Part model, mm, in its own coordinate system. Face numbers are marked on the shaded views. Round coordinates to 2 decimals unless told otherwise and drop trailing zeros. Write each loop counter-clockwise with the first axis right and the second up, starting at its lowest first coordinate (ties: lowest second). Pieces come first, ordered by that corner, then holes.
```python
from build123d import *

# Parameters (mm, degrees)
SKETCH_1_W          = 72
SKETCH_1_H          = 99.6
SKETCH_1_R          = 1.6
EXTRUDE_1_DEPTH     = 2
FILLET_1_R          = 3
SKETCH_7_W          = 2.173613934
SKETCH_7_H          = 4.368539476
CUT_EXTRUDE_1_DEPTH = 10
CUT_EXTRUDE_2_DEPTH = 10
FILLET_2_R          = 2
SKETCH_9_W          = 2.173613934
SKETCH_9_H          = 2.184269738
EXTRUDE_5_DEPTH     = 2
FILLET_4_R          = 2
FILLET_5_R          = 2
EXTRUDE_4_DEPTH     = 5


with BuildPart() as part:
    # Sketch 1 → Extrude 1 (new body)
    with BuildSketch(Plane(origin=(0, 0, 0), x_dir=(1, 0, 0), z_dir=(0, 1, 0))):
        with Locations((36, -49.8)):
            Rectangle(SKETCH_1_W, SKETCH_1_H)
        with Locations(Location((11, -5, 0), (0, 0, 270))):
            Circle(SKETCH_1_R, mode=Mode.SUBTRACT)
        with Locations(Location((14, -95, 0), (0, 0, 270))):
            Circle(SKETCH_1_R, mode=Mode.SUBTRACT)
        with Locations(Location((58, -95, 0), (0, 0, 90))):
            Circle(SKETCH_1_R, mode=Mode.SUBTRACT)
        with Locations(Location((61, -5, 0), (0, 0, 90))):
            Circle(SKETCH_1_R, mode=Mode.SUBTRACT)
        with Locations(Location((2.31, -58.92, 0), (0, 0, 270))):
            Circle(SKETCH_1_R, mode=Mode.SUBTRACT)
        with Locations(Location((69.69, -58.92, 0), (0, 0, 90))):
            Circle(SKETCH_1_R, mode=Mode.SUBTRACT)
    extrude(amount=EXTRUDE_1_DEPTH)

    # Fillet 1
    fillet_1_edges = [part.edges().sort_by_distance(p)[0] for p in [
        (0, 1, 0),
        (72, 1, 0),
        (72, 1, 99.6),
        (0, 1, 99.6),
    ]]
    fillet(fillet_1_edges, radius=FILLET_1_R)

    # Sketch 7 → Cut-Extrude 1 (cut)
    with BuildSketch(Plane(origin=(0, 2, 0), x_dir=(1, 0, 0), z_dir=(0, 1, 0))):
        with Locations((36, -99.6)):
            Rectangle(SKETCH_7_W, SKETCH_7_H)
    extrude(amount=-CUT_EXTRUDE_1_DEPTH, mode=Mode.SUBTRACT)

    # Sketch 8 → Cut-Extrude 2 (cut)
    with BuildSketch(Plane(origin=(0, 2, 0), x_dir=(1, 0, 0), z_dir=(0, 1, 0))):
        with BuildLine():
            Line((3, -99.6), (3, -79.6))
            Line((3, -79.6), (0, -79.6))
            Line((0, -79.6), (0, -96.6))
            ThreePointArc((0, -96.6), (0.878679656, -98.721320344), (3, -99.6))
        make_face()
        with BuildLine():
            ThreePointArc((72, -96.6), (71.121320344, -98.721320344), (69, -99.6))
            Line((69, -99.6), (69, -79.6))
            Line((69, -79.6), (72, -79.6))
            Line((72, -79.6), (72, -96.6))
        make_face()
        with BuildLine():
            ThreePointArc((3, 0), (0.878679656, -0.878679656), (0, -3))
            Line((0, -3), (0, -18))
            Line((0, -18), (3, -18))
            Line((3, -18), (3, 0))
        make_face()
    cut_extrude_2 = extrude(amount=-CUT_EXTRUDE_2_DEPTH, mode=Mode.SUBTRACT)

    # Fillet 2
    fillet_2_edges = [part.edges().sort_by_distance(p)[0] for p in [
        (69, 1, 79.6),
        (3, 1, 79.6),
    ]]
    fillet(fillet_2_edges, radius=FILLET_2_R)

    # Mirror 2: Cut-Extrude 2 across plane
    add(cut_extrude_2.mirror(Plane(origin=(36, 0, 0), x_dir=(0, 0, 1), z_dir=(1, 0, 0))), mode=Mode.SUBTRACT)

    # Sketch 9 → Extrude 5 (add)
    with BuildSketch(Plane(origin=(0, 2, 0), x_dir=(1, 0, 0), z_dir=(0, 1, 0))):
        with Locations((36, -98.507865131)):
            Rectangle(SKETCH_9_W, SKETCH_9_H)
    extrude(amount=-EXTRUDE_5_DEPTH)

    # Fillet 4
    fillet_4_edges = [part.edges().sort_by_distance(p)[0] for p in [
        (69, 1, 18),
        (3, 1, 18),
    ]]
    fillet(fillet_4_edges, radius=FILLET_4_R)

    # Fillet 5
    fillet_5_edges = [part.edges().sort_by_distance(p)[0] for p in [
        (3, 1, 79.6),
        (69, 1, 79.6),
    ]]
    fillet(fillet_5_edges, radius=FILLET_5_R)


with BuildPart() as body_2:
    # Sketch 6 → Extrude 4 (new body)
    with BuildSketch(Plane(origin=(0, -3, 0), x_dir=(-1, 0, 0), z_dir=(0, -1, 0))):
        with BuildLine():
            Line((-2, 4), (-70, 4))
            ThreePointArc((-70, 4), (-74.242640687, 2.242640687), (-76, -2))
            Line((-76, -2), (-76, -18))
            Line((-76, -18), (-76, -97.6))
            ThreePointArc((-76, -97.6), (-74.242640687, -101.842640687), (-70, -103.6))
            Line((-70, -103.6), (-2, -103.6))
            ThreePointArc((-2, -103.6), (2.242640687, -101.842640687), (4, -97.6))
            Line((4, -97.6), (4, -4))
            ThreePointArc((4, -4), (3.146700168, 1.610025126), (-2, 4))
        make_face()
    extrude(amount=-EXTRUDE_4_DEPTH)

    # Combine 1: cut part
    add(part.part, mode=Mode.SUBTRACT)


solid = body_2.part
```
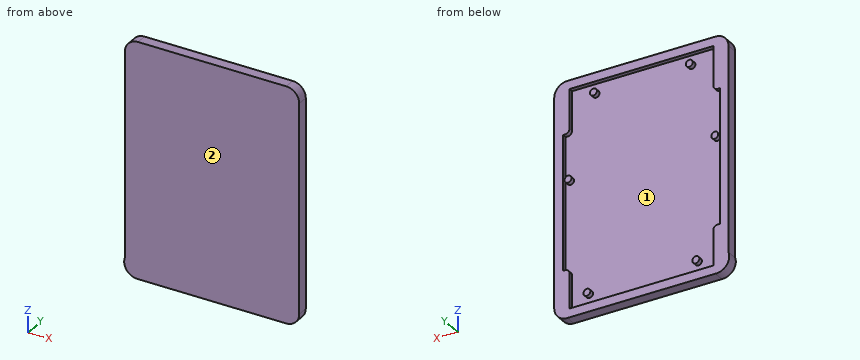
Q1. Cut at C-C on x = 14. Write the cut outline in (y, z), plus the area to 3 significant figures.
Values follow:
outline: (-3, -4) - (2, -4) - (2, 0) - (0, 0) - (0, 93.4) - (2, 93.4) - (2, 96.6) - (0, 96.6) - (0, 99.6) - (2, 99.6) - (2, 103.6) - (-3, 103.6) - close
area: 345 mm2
Q2. Drop flat-ended pins along their axis: pin 1 (2.5 mm diameter, centred on y = 0.5, z = 56.5, fed in from -X); pin 2 (0.5 mm diameter, centred on x = 0.5, y = 1, fed in from +Z); pin 3 (1 mm diameter, centred on x = 34.5, y = 1, fed in from -Z). Give the stop position or say it passes through.
Values follow:
pin 1: stops at x = -4
pin 2: stops at z = 103.47
pin 3: stops at z = -4
Q3. Cut at A-A on y = 0.9. State how many separate pieces and enclosed holes the cut face has, plus the area to 3 significant figures.
Values follow:
separate pieces: 7
enclosed holes: 1
area: 1,680 mm2
Q4. Cut at B-B on z = 58.92. Write the cut outline in (x, y).
Values follow:
outline: (-4, -3) - (76, -3) - (76, 2) - (72, 2) - (72, 0) - (71.29, 0) - (71.29, 2) - (68.09, 2) - (68.09, 0) - (3.91, 0) - (3.91, 2) - (0.71, 2) - (0.71, 0) - (0, 0) - (0, 2) - (-4, 2) - close
Q5. Cut at D-D on z = 12. Write the cut outline in (x, y).
Values follow:
outline: (-4, -3) - (76, -3) - (76, 2) - (69, 2) - (69, 0) - (3, 0) - (3, 2) - (-4, 2) - close
Q6. Mould opens along Z. For the marked faces 1 and 2 say: +Z half, -Z half, draft (parallel to the pull), parting line (faces both ways), or undercut.
Values follow:
face 1: undercut
face 2: draft
Q7. Wall check: L1, parallel to Z at x = 48, y = 0.75; L2, parallel to X at y = 0.75, z = 77; L3, parallel to X at y = -0.5, z = 24.5. Give the ranges that are in metal, low to high.
Values follow:
L1: z = -4 to 0, 99.6 to 103.6
L2: x = -4 to 0, 72 to 76
L3: x = -4 to 76
